Read the model definition and answer for the solid it produces. Units are mm, in the model's axes. A direction names the side the tool comes from. Give positions to 0.01 mm unless a question says otherwise; leave off trailing zeros. Loops run counter-clockwise (first coordinate to the right, second up) from the corner with the lowest first, then second, coordinate; pieces in that order, holes last. Notation, with made-up numbers: (-2.75, 68) - (32.25, 68) arc R21 cw to (32.25, 90) - close; hole circle Ø5 at (63, 88.25). An arc over 180 degrees is marked (long way). Write item = value, one per line. Start each with the question number.
from build123d import *

# Parameters (mm, degrees)
SCHIZZO1_W                                           = 65
SCHIZZO1_H                                           = 235
ESTRUSIONE_ESTRUSIONE1_DEPTH                         = 16
SCHIZZO2_W                                           = 10
SCHIZZO2_H                                           = 37
TAGLIO_ESTRUSIONE1_DEPTH                             = 239.105018847
SCHIZZO3_W                                           = 33
SCHIZZO3_H                                           = 90
TAGLIO_ESTRUSIONE2_DEPTH                             = 239.432380351
SCHIZZO4_W                                           = 10
SCHIZZO4_H                                           = 22
TAGLIO_ESTRUSIONE3_DEPTH                             = 239.105018847
FORO_LAMATO_PER_VITE_M4_A_TESTA_ESAGONAL_D           = 4.5
FORO_LAMATO_PER_VITE_M4_A_TESTA_ESAGONAL_CBORE_D     = 8
FORO_LAMATO_PER_VITE_M4_A_TESTA_ESAGONAL_CBORE_DEPTH = 4
RACCORDO1_R                                          = 2
RACCORDO2_R                                          = 4
RACCORDO3_R                                          = 6
FORO_PER_VITE_M4_1_D                                 = 4.5
FORO_PER_VITE_M4_1_DEPTH                             = 188
FORO_PER_VITE_M4_1_TIP                               = 1.351936393
SCHIZZO10_W                                          = 3
SCHIZZO10_H                                          = 15
ESTRUSIONE_ESTRUSIONE2_DEPTH                         = 15
SCHIZZO11_R                                          = 2.5
TAGLIO_ESTRUSIONE4_DEPTH                             = 10
SMUSSO1_SIZE                                         = 8


with BuildPart() as part:
    # Schizzo1 → Estrusione-Estrusione1 (new body)
    with BuildSketch(Plane(origin=(6, 0, 0), x_dir=(0, 0, -1), z_dir=(1, 0, 0))):
        with Locations((4.5, 117.5)):
            Rectangle(SCHIZZO1_W, SCHIZZO1_H)
    extrude(amount=-ESTRUSIONE_ESTRUSIONE1_DEPTH)

    # Schizzo2 → Taglio-Estrusione1 (cut, through all)
    with BuildSketch(Plane.XZ):
        with Locations((-5, -18.5)):
            Rectangle(SCHIZZO2_W, SCHIZZO2_H)
    extrude(amount=-TAGLIO_ESTRUSIONE1_DEPTH, mode=Mode.SUBTRACT)

    # Schizzo3 → Taglio-Estrusione2 (cut, through all)
    with BuildSketch(Plane(origin=(6, 0, 0), x_dir=(0, 0, -1), z_dir=(1, 0, 0))):
        with Locations((20.5, 45)):
            Rectangle(SCHIZZO3_W, SCHIZZO3_H)
    extrude(amount=-TAGLIO_ESTRUSIONE2_DEPTH, mode=Mode.SUBTRACT)

    # Schizzo4 → Taglio-Estrusione3 (cut, through all)
    with BuildSketch(Plane.XZ):
        with Locations((1, 17)):
            Rectangle(SCHIZZO4_W, SCHIZZO4_H)
    extrude(amount=-TAGLIO_ESTRUSIONE3_DEPTH, mode=Mode.SUBTRACT)

    # Foro lamato per Vite M4 a testa esagonale-1 (through all)
    with Locations(Plane.ZY):
        with Locations((-17.5, 175), (-17.5, 155), (-17.5, 135)):
            CounterBoreHole(FORO_LAMATO_PER_VITE_M4_A_TESTA_ESAGONAL_D / 2, FORO_LAMATO_PER_VITE_M4_A_TESTA_ESAGONAL_CBORE_D / 2, FORO_LAMATO_PER_VITE_M4_A_TESTA_ESAGONAL_CBORE_DEPTH)

    # Raccordo1
    raccordo1_edges = [part.edges().sort_by_distance(p)[0] for p in [
        (0, 117.5, 0),
        (-4, 117.5, 6),
    ]]
    fillet(raccordo1_edges, radius=RACCORDO1_R)

    # Raccordo2
    raccordo2_edges = [part.edges().sort_by_distance(p)[0] for p in [
        (-10, 117.5, 0),
        (6, 117.5, 6),
    ]]
    fillet(raccordo2_edges, radius=RACCORDO2_R)

    # Raccordo3
    raccordo3_edges = [part.edges().sort_by_distance(p)[0] for p in [
        (3, 90, -4),
    ]]
    fillet(raccordo3_edges, radius=RACCORDO3_R)

    # Foro per Vite M4-1
    with Locations(Plane(origin=(-4, 0, 0), x_dir=(0, 0, -1), z_dir=(1, 0, 0))):
        with Locations((-23, 7), (-13, 7)):
            Hole(FORO_PER_VITE_M4_1_D / 2, depth=FORO_PER_VITE_M4_1_DEPTH)
            with Locations((0, 0, -(FORO_PER_VITE_M4_1_DEPTH + FORO_PER_VITE_M4_1_TIP / 2))):  # 118° drill point
                Cone(0, FORO_PER_VITE_M4_1_D / 2, FORO_PER_VITE_M4_1_TIP, mode=Mode.SUBTRACT)

    # Schizzo10 → Estrusione-Estrusione2 (add)
    with BuildSketch(Plane.ZY.offset(10)):
        with Locations((13.5, 117.5)):
            Rectangle(SCHIZZO10_W, SCHIZZO10_H)
    extrude(amount=ESTRUSIONE_ESTRUSIONE2_DEPTH)

    # Schizzo11 → Taglio-Estrusione4 (cut)
    with BuildSketch(Plane.ZY.offset(10)):
        with Locations((19, 117.5)):
            Circle(SCHIZZO11_R)
    extrude(amount=-TAGLIO_ESTRUSIONE4_DEPTH, mode=Mode.SUBTRACT)

    # Smusso1
    smusso1_edges = [part.edges().sort_by_distance(p)[0] for p in [
        (-10, 117.5, 12),
    ]]
    chamfer(smusso1_edges, length=SMUSSO1_SIZE - 0.0001)  # a hair under: the kernel refuses the full size


solid = part.part
1. A tool of negligible diameter and unlimited length cuts with its end or side. For faces 1 (the cylindrical face through (-7, 120, 19)), 2 (the flat face through (4, 153, -16)), 3 (the flat face through (0, 168, -20)), 4 (the flat face through (3, 41, -4)), from which of +Z, -Z, +X, -X, +Y, -Y can it reach the whole face along a straight path? Write none if from no direction.
2. For a pull along Z with two mould halves and no side action, classify faces 5 (the flat face through (-21, 117, 12)), 6 (the cylindrical face through (5.014, 133.004, -18.538)), 7 (the flat face through (-16, 125, 12)), 8 (the flat face through (-7, 116, 28)) as released by +Z, released by -Z, zero draft, split by the parting line, or undercut.
3. Consider line 1 along Y through (x, z) = (2.3, -17.5); line 2 along Y through (x, z) = (5.3, -17.5); line 3 along Y through (x, z) = (-8, 23). Determine where each line is inside the solid, lowest interval first. Write a range as [from, to].
4. A cutting plane is placed at A-A on z = -17.5. Give the vertices of the cut face in (x, y).
5. Given P1, Ø7.5, axis at x = -16, y = 120, coming from the +Z side; P2, Ø1.5, axis at x = 0.5, y = 30.5, coming from the -Z side; P3, Ø3.5, axis at x = -17.5, z = 11.5, coming from the +Y side; P4, Ø3, axis at x = -10.5, y = 151, coming from the +Z side, each flat-ended and moving along its own axis, determine where each tip first touches the part or whether it passes through.
6. A cutting plane is placed at D-D on x = -12.5. Give the vertices of the cut face in (y, z), and give its area (3 significant figures).
7. A cutting plane is placed at B-B on y = 7. Give the vertices of the cut face in (x, z), and give its area (3 significant figures).
Reply:
q1.face_1 = +X, -X
q1.face_2 = -X
q1.face_3 = -Z, -X, +Y, -Y
q1.face_4 = -Z, +X, -X, -Y
q2.face_5 = released by -Z
q2.face_6 = undercut
q2.face_7 = zero draft
q2.face_8 = released by +Z
q3.line_1 = [90, 131], [139, 151], [159, 171], [179, 235]
q3.line_2 = [90, 132.75], [137.25, 152.75], [157.25, 172.75], [177.25, 235]
q3.line_3 = [0, 4.75], [9.25, 235]
q4.outline = (0, 90) - (6, 90) - (6, 132.75) - (4, 132.75) - (4, 131) - (0, 131) - close; (0, 139) - (4, 139) - (4, 137.25) - (6, 137.25) - (6, 152.75) - (4, 152.75) - (4, 151) - (0, 151) - close; (0, 159) - (4, 159) - (4, 157.25) - (6, 157.25) - (6, 172.75) - (4, 172.75) - (4, 171) - (0, 171) - close; (0, 179) - (4, 179) - (4, 177.25) - (6, 177.25) - (6, 235) - (0, 235) - close
q5.P1 = 15
q5.P2 = -4
q5.P3 = 125
q5.P4 = 28
q6.outline = (110, 6.5) - (125, 6.5) - (125, 15) - (110, 15) - close
q6.area = 127 mm^2
q7.outline = (-10, 4) arc R4 ccw to (-6, 0) - (-2, 0) arc R2 cw to (0, -2) - (0, -4) - (6, -4) - (6, 2) arc R4 ccw to (2, 6) - (-2, 6) arc R2 cw to (-4, 8) - (-4, 10.75) - (-10, 10.75) - close; (-10, 15.25) - (-4, 15.25) - (-4, 20.75) - (-10, 20.75) - close; (-10, 25.25) - (-4, 25.25) - (-4, 28) - (-10, 28) - close
q7.area = 193 mm^2
